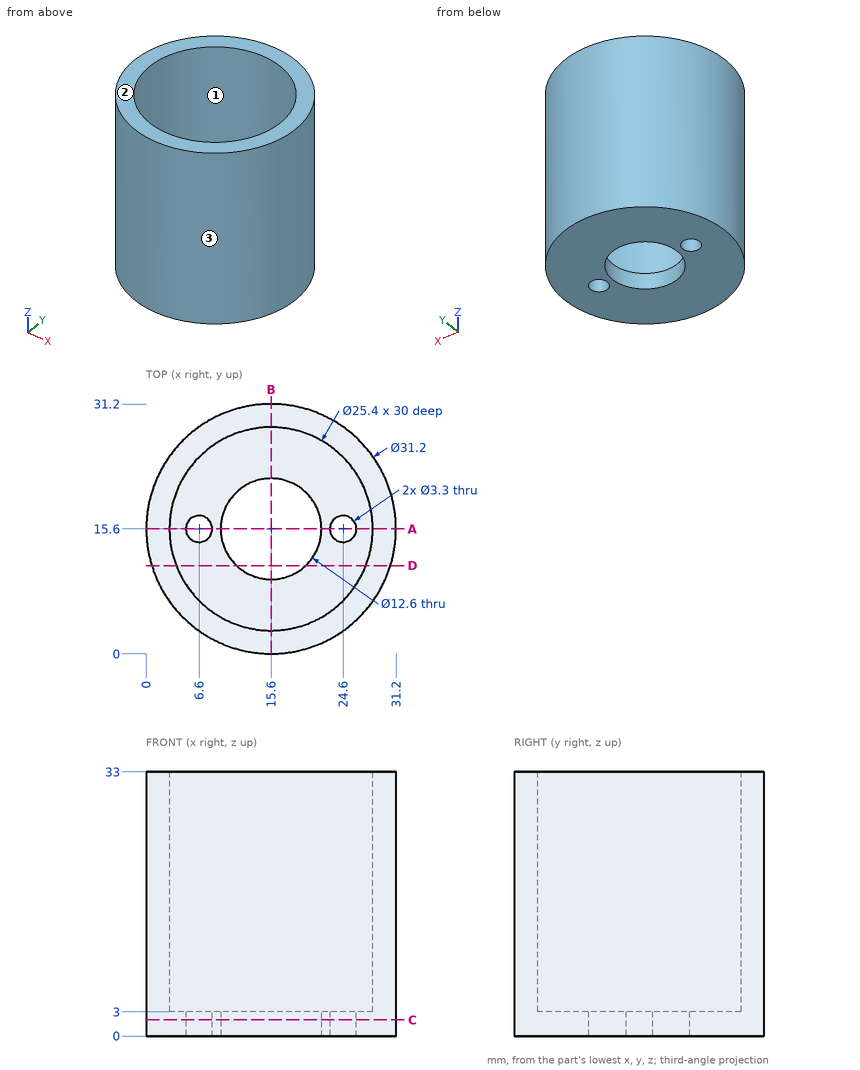
For this review, use the dimensioned drawing (mm, ordinates from the lowest corner) and the shaded views. Round coordinates to 2 decimals unless told otherwise and drop trailing zeros. Order: outer loops, then holes, each group sorted by start corner. A loop starts at its lowest first (then second) coordinate and runs counter-clockwise, first axis right, second up. Notation, with made-up numbers: (88, 34) -> (146, 34) arc R11 ccw to (146, 43) -> close; hole circle Ø1 at (64.5, -25). An arc over 180 degrees is marked (long way). Use CSV: the item, a comma, the result in double quotes. Start each with the question number.
(1) Mouldability with a two-part tool opening along Y and no side actions: class the marked faces 1, 2 and 3 as pulls with the +Y half, pulls with the -Y half, needs draft (parallel to the pull), parting line crosses it, or undercut.
(2) Insertion check: pin 1 (2 mm diameter, centred on x = 25.5, z = 21.5, fed in from -Y); pin 2 (8 mm diameter, centred on y = 6, z = 28.5, fed in from +X); pin 3 (1.5 mm diameter, centred on x = 11.5, z = 25.5, fed in from -Y); pin 4 (2 mm diameter, centred on x = 24.6, y = 15.6, fed in from +Z). Each pin has a flat end and moves straight along its axis. Give the tip position at first contact, or say it passes through.
(3) Consider section B-B on x = 15.6. Write out the cut boundary in (y, z).
(4) Consider section D-D on y = 11. Write out the cut boundary in (x, z), and give its area (3 significant figures).
(5) Consider section C-C on z = 2. Write out the cut boundary in (x, y).
(6) Consider section A-A on y = 15.6. Write out the cut boundary in (x, z), and give its area (3 significant figures).
(7) Wall thickness on probe 1 along Y at (x, z) = (15.6, 21); probe 2 along Z at (x, y) = (5.5, 8.5); probe 3 along Y at (x, z) = (10, 22.5): over which ranges is each line inside the solid? List them lowest first. Write a range as from..to.
Responses:
1,face 1,"undercut"
1,face 2,"needs draft"
1,face 3,"parting line crosses it"
2,pin 1,"y = 2.79"
2,pin 2,"x = 30.16"
2,pin 3,"y = 0.36"
2,pin 4,"through"
3,outline,"(0, 0) -> (9.3, 0) -> (9.3, 3) -> (2.9, 3) -> (2.9, 33) -> (0, 33) -> close; (21.9, 0) -> (31.2, 0) -> (31.2, 33) -> (28.3, 33) -> (28.3, 3) -> (21.9, 3) -> close"
4,outline,"(0.69, 0) -> (11.3, 0) -> (11.3, 3) -> (3.76, 3) -> (3.76, 33) -> (0.69, 33) -> close; (19.9, 0) -> (30.51, 0) -> (30.51, 33) -> (27.44, 33) -> (27.44, 3) -> (19.9, 3) -> close"
4,area,"248 mm²"
5,outline,"circle Ø31.2 at (15.6, 15.6); hole circle Ø3.3 at (6.6, 15.6); hole circle Ø12.6 at (15.6, 15.6); hole circle Ø3.3 at (24.6, 15.6)"
6,outline,"(0, 0) -> (4.95, 0) -> (4.95, 3) -> (2.9, 3) -> (2.9, 33) -> (0, 33) -> close; (8.25, 0) -> (9.3, 0) -> (9.3, 3) -> (8.25, 3) -> close; (21.9, 0) -> (22.95, 0) -> (22.95, 3) -> (21.9, 3) -> close; (26.25, 0) -> (31.2, 0) -> (31.2, 33) -> (28.3, 33) -> (28.3, 3) -> (26.25, 3) -> close"
6,area,"210 mm²"
7,probe 1,"0..2.9, 28.3..31.2"
7,probe 2,"0..3"
7,probe 3,"1.04..4.2, 27..30.16"
